```python
from build123d import *

# Parameters (mm, degrees)
SKETCH2_R          = 1.25
CUT_EXTRUDE1_DEPTH = 4


with BuildPart() as part:
    # Sketch1 → Revolve1 (revolve)
    with BuildSketch(Plane.XY, mode=Mode.PRIVATE) as revolve1_sk:
        Polygon((0, 0), (0, 3), (-0.5, 3), (-0.5, 5.5), (-5, 5.5), (-5, 33), (-7.5, 33), (-7.5, 33.75), (-21, 33.75), (-21, 22), (-25, 22), (-25, 18), (-27, 18), (-27, 17), (-30.5, 17), (-30.5, 0), align=None)
    revolve(revolve1_sk.sketch.rotate(Axis((-34.008884984, 0, 0), (1, 0, 0)), 90), axis=Axis((-34.008884984, 0, 0), (1, 0, 0)))

    # Sketch2 → Cut-Extrude1 (cut)
    with BuildSketch(Plane.ZY.offset(25)):
        with Locations((-7.749339505, 18.708560533)):
            Circle(SKETCH2_R)
        with Locations((7.749339505, 18.708560533)):
            Circle(SKETCH2_R)
        with Locations((18.708560533, 7.749339505)):
            Circle(SKETCH2_R)
        with Locations((18.708560533, -7.749339505)):
            Circle(SKETCH2_R)
        with Locations((7.749339505, -18.708560533)):
            Circle(SKETCH2_R)
        with Locations((-7.749339505, -18.708560533)):
            Circle(SKETCH2_R)
        with Locations((-18.708560533, -7.749339505)):
            Circle(SKETCH2_R)
        with Locations((-18.708560533, 7.749339505)):
            Circle(SKETCH2_R)
    extrude(amount=-CUT_EXTRUDE1_DEPTH, mode=Mode.SUBTRACT)


solid = part.part
```
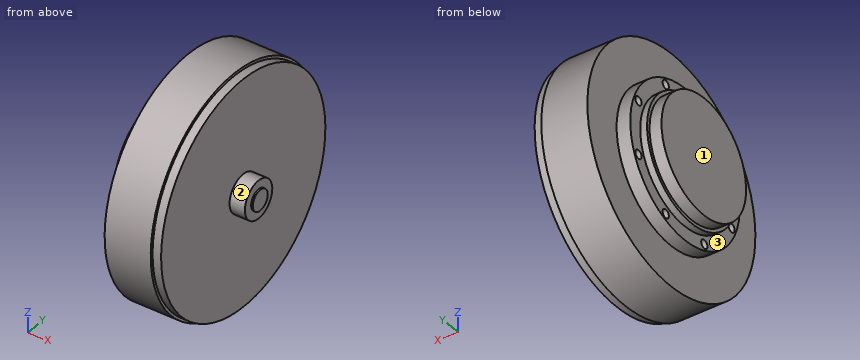
Design review of the part built by this model. Coordinates are the model's own, in mm. Face numbers are marked on the shaded views. A direction names the side the tool comes from. Give positions to 0.01 mm unless a question says otherwise; leave off trailing zeros. Write each loop counter-clockwise with the first axis right and the second up, starting at its lowest first coordinate (ties: lowest second). Pieces come first, ordered by that corner, then holes. Notation, with made-up numbers: (78, 3) -> (132, 3) arc R16 cw to (132, 23) -> close; hole circle Ø8 at (-3.75, 55.25). An arc over 180 degrees is marked (long way). Answer in a Markdown table with one row per item.
(1) For the marked faces 1, 2 and 3, list the 3-axis set-ups (+Z, -Z, +X, -X, +Y, -Y) from which the entire face can be reached by the end or side of a thin tool; tool diameter is ignored.
Results:
| item | result |
|---|---|
| face 1 | +Z, -Z, -X, +Y, -Y |
| face 2 | +X |
| face 3 | -X |
(2) Consider section A-A (y = 0). State the section outline as (x, z) points, then the cut area to 3 significant figures.
Results:
| item | result |
|---|---|
| outline | (-30.5, -17) -> (-27, -17) -> (-27, -18) -> (-25, -18) -> (-25, -22) -> (-21, -22) -> (-21, -33.75) -> (-7.5, -33.75) -> (-7.5, -33) -> (-5, -33) -> (-5, -5.5) -> (-0.5, -5.5) -> (-0.5, -3) -> (0, -3) -> (0, 3) -> (-0.5, 3) -> (-0.5, 5.5) -> (-5, 5.5) -> (-5, 33) -> (-7.5, 33) -> (-7.5, 33.75) -> (-21, 33.75) -> (-21, 22) -> (-25, 22) -> (-25, 18) -> (-27, 18) -> (-27, 17) -> (-30.5, 17) -> close |
| area | 1,500 mm2 |
(3) Clearance check with flat-ended pins moving along their axes: pin 1 (3 mm diameter, centred on y = 7.75, z = 18.71, fed in from -X); pin 2 (20 mm diameter, centred on y = 14, z = 11.5, fed in from +X); pin 3 (1.2 mm diameter, centred on y = -19, z = -8, fed in from -X); pin 4 (2 mm diameter, centred on x = -26.5, y = 24, fed in from +Z). State where each tip first meets the part, or that it passes through.
Results:
| item | result |
|---|---|
| pin 1 | x = -25 |
| pin 2 | x = -5 |
| pin 3 | x = -21 |
| pin 4 | through |
(4) To check wall thickness, follow probe 1 along X at (y, z) = (14.5, -26.5); probe 2 along X at (y, z) = (12.5, 8); probe 3 along Y at (x, z) = (-14, 1). State the ranges of each line that lie inside material, in increasing order.
Results:
| item | result |
|---|---|
| probe 1 | -21 to -5 |
| probe 2 | -30.5 to -5 |
| probe 3 | -33.74 to 33.74 |
(5) Consider section C-C (x = -28). State the section outline as (y, z) points, then the cut area to 3 significant figures.
Results:
| item | result |
|---|---|
| outline | circle Ø34 at (0, 0) |
| area | 908 mm2 |
(6) Consider section D-D (y = 24). State the section outline as (x, z) points, then the cut area to 3 significant figures.
Results:
| item | result |
|---|---|
| outline | (-21, -23.73) -> (-7.5, -23.73) -> (-7.5, -22.65) -> (-5, -22.65) -> (-5, 22.65) -> (-7.5, 22.65) -> (-7.5, 23.73) -> (-21, 23.73) -> close |
| area | 754 mm2 |
